Source: CAD feature listing. Evaluate the final solid. Frame: model axes, mm. Give positions to 0.01 mm unless a question says otherwise; leave off trailing zeros. Order: outer loops, then holes, each group sorted by start corner. A loop starts at its lowest first (then second) coordinate and runs counter-clockwise, first axis right, second up. Notation, with made-up numbers: (-29, 53.5) -> (-1, 53.5) arc R16 cw to (-1, 67.5) -> close; hole circle Ø9 at (33, 48.25). An arc over 180 degrees is marked (long way). Answer in a Markdown table with one row per item.
```python
from build123d import *

# Parameters (mm, degrees)
SKETCH1_W           = 25.4
SKETCH1_H           = 63.5
BOSS_EXTRUDE2_DEPTH = 6.35
SKETCH3_R           = 2.778125
CUT_EXTRUDE1_DEPTH  = 69.685751798


with BuildPart() as part:
    # Sketch1 → Boss-Extrude2 (new body)
    with BuildSketch(Plane(origin=(0, 0, 0), x_dir=(1, 0, 0), z_dir=(0, 1, 0))):
        with Locations((-12.7, 31.75)):
            Rectangle(SKETCH1_W, SKETCH1_H)
    extrude(amount=-BOSS_EXTRUDE2_DEPTH)

    # Sketch3 → Cut-Extrude1 (cut, through all)
    with BuildSketch(Plane(origin=(0, 0, 0), x_dir=(1, 0, 0), z_dir=(0, 1, 0))):
        with Locations(Location((-12.7, 21.166666667, 0), (0, 0, 270))):
            Circle(SKETCH3_R)
        with Locations(Location((-12.7, 42.333333333, 0), (0, 0, 270))):
            Circle(SKETCH3_R)
    extrude(amount=-CUT_EXTRUDE1_DEPTH, mode=Mode.SUBTRACT)


solid = part.part
```
(1) Section query A-A (x = -12.7). Return the cut outline in (y, z).
A:
| item | result |
|---|---|
| outline | (-6.35, -63.5) -> (0, -63.5) -> (0, -45.11) -> (-6.35, -45.11) -> close; (-6.35, -39.56) -> (0, -39.56) -> (0, -23.94) -> (-6.35, -23.94) -> close; (-6.35, -18.39) -> (0, -18.39) -> (0, 0) -> (-6.35, 0) -> close |
(2) Section query B-B (y = -2.25). Return the cut outline in (x, z), plus the area to 3 significant figures.
A:
| item | result |
|---|---|
| outline | (-25.4, -63.5) -> (0, -63.5) -> (0, 0) -> (-25.4, 0) -> close; hole circle Ø5.56 at (-12.7, -42.33); hole circle Ø5.56 at (-12.7, -21.17) |
| area | 1,560 mm^2 |
(3) Pull-direction query (Z, two-part tool) for faces 1 (the flat face through (-25.4, -3, -31)), 2 (the cylindrical face through (-13.764, -3.131, -39.767)), 3 (the flat face through (-13, -3, -63.5)); classes: +Z half, -Z half, draft (parallel to the pull), parting line (faces both ways), or undercut.
A:
| item | result |
|---|---|
| face 1 | draft |
| face 2 | undercut |
| face 3 | -Z half |
(4) Ray query, probe 1 along Z at (x, y) = (-15, -5); probe 2 along X at (y, z) = (-6, -21); probe 3 along X at (y, z) = (-3.25, -43). Return the intervals inside material, ascending.
A:
| item | result |
|---|---|
| probe 1 | z = -63.5 to -43.89, -40.78 to -22.72, -19.61 to 0 |
| probe 2 | x = -25.4 to -15.47, -9.93 to 0 |
| probe 3 | x = -25.4 to -15.4, -10 to 0 |
